CAD build for the part. Positions are in the model's coordinates, mm. A direction names the side the tool comes from. Round coordinates to 2 decimals unless told otherwise and drop trailing zeros. Order: outer loops, then holes, each group sorted by start corner. A loop starts at its lowest first (then second) coordinate and runs counter-clockwise, first axis right, second up. Notation, with made-up numbers: (8, 68) - (17, 68) arc R15 ccw to (17, 97) - close; hole circle Ø2 at (66.25, -9.75). An arc over 180 degrees is marked (long way). Write item = value, one per line.
from build123d import *

# Parameters (mm, degrees)
BLANKSKE_W          = 60
BLANKSKE_H          = 12.5
BLANK_DEPTH         = 6
TOOTHCUTSIM_DEPTH   = 62.581247146
TEETHCUTS_COUNT     = 39
TEETHCUTS_PITCH     = 1.570796325
SKETCH1_W           = 60
SKETCH1_H           = 6
BOSS_EXTRUDE1_DEPTH = 10
SKETCH4_W           = 88.884112985
SKETCH4_H           = 15.47203355
CUT_EXTRUDE3_DEPTH  = 62.581247146
SKETCH3_W           = 50
SKETCH3_H           = 5.375
CUT_EXTRUDE2_DEPTH  = 10
FILLET3_R           = 5


with BuildPart() as part:
    # BlankSke → Blank (new body)
    with BuildSketch(Plane.XY):
        with Locations((30, 6.25)):
            Rectangle(BLANKSKE_W, BLANKSKE_H)
    extrude(amount=-BLANK_DEPTH)

    # TooCutSkeSim → ToothCutSim (cut, through all)
    with BuildSketch(Plane.XY):
        Polygon((0.222217685, 11.375), (-0.222217685, 11.375), (-0.640929042, 12.5254), (0.640929042, 12.5254), align=None)
    toothcutsim = extrude(amount=-TOOTHCUTSIM_DEPTH, mode=Mode.SUBTRACT)

    # TeethCuts: ToothCutSim ×39
    with Locations(*[(i * TEETHCUTS_PITCH, 0, 0) for i in range(1, TEETHCUTS_COUNT)]):
        add(toothcutsim, mode=Mode.SUBTRACT)

    # Sketch1 → Boss-Extrude1 (add)
    with BuildSketch(Plane.XZ):
        with Locations((30, -3)):
            Rectangle(SKETCH1_W, SKETCH1_H)
    extrude(amount=BOSS_EXTRUDE1_DEPTH)

    # Sketch4 → Cut-Extrude3 (cut, through all)
    with BuildSketch(Plane.XY):
        with Locations((41.448981395, -7.736016775)):
            Rectangle(SKETCH4_W, SKETCH4_H)
    extrude(amount=-CUT_EXTRUDE3_DEPTH, mode=Mode.SUBTRACT)

    # Sketch3 → Cut-Extrude2 (cut)
    with BuildSketch(Plane.XY):
        with Locations((30, 5.6875)):
            Rectangle(SKETCH3_W, SKETCH3_H)
    extrude(amount=-CUT_EXTRUDE2_DEPTH, mode=Mode.SUBTRACT)

    # Fillet3
    fillet3_edges = [part.edges().sort_by_distance(p)[0] for p in [
        (0, 0, -3),
        (60, 0, -3),
    ]]
    fillet(fillet3_edges, radius=FILLET3_R)


solid = part.part
(1) Pull direction Y, two halves, no side cores. Call faces 1 (the flat face through (55, 6, -3)), 2 (the flat face through (30, 3, -3)), 3 (the flat face through (23.138, 11.93, -2.958)): released by +Y, released by -Y, zero draft, split by the parting line, or undercut.
Solved:
face_1 = undercut
face_2 = undercut
face_3 = released by +Y
(2) Band-saw the part on A-A on y = 3.5. List the corners of the cut face in (x, z).
Solved:
outline = (0.23, -6) - (5, -6) - (5, 0) - (0.23, 0) - close; (55, -6) - (59.77, -6) - (59.77, 0) - (55, 0) - close
(3) Probe line 1 along X through (y, z) = (6.5, -1.75); line 2 along Y through (x, z) = (11, -1.3) (3 decimals); line 3 along Y through (x, z) = (49.5, -3.5) (3 decimals). List the from-to ranges inside material, lowest first.
Solved:
line_1 = 0 to 5, 55 to 60
line_2 = 0 to 3, 8.375 to 11.375
line_3 = 0 to 3, 8.375 to 12.5
(4) Tool access for faces 4 (the flat face through (16.855, 11.93, -2.958)), 5 (the flat face through (0.43, 11.95, -2.96)): list every direction of +Z, -Z, +X, -X, +Y, -Y with a clear straight run to the whole face (end or side of a thin tool).
Solved:
face_4 = +Z, -Z, +Y
face_5 = +Z, -Z, -X, +Y
(5) Drop a flat-ended pin along its axis: pin 1 (3 mm diameter, centred on x = 28, y = 5.5, fed in from -Z) (3 decimals). Give the stop position or say it passes through.
Solved:
pin_1 = through
